Source: CAD feature listing. Evaluate the final solid. Frame: model axes, mm. Face numbers are marked on the shaded views. A direction names the side the tool comes from. Give positions to 0.01 mm unless a question says otherwise; leave off trailing zeros. Order: outer loops, then holes, each group sorted by start corner. A loop starts at its lowest first (then second) coordinate and runs counter-clockwise, first axis right, second up.
from build123d import *

# Parameters (mm, degrees)
SKETCH_1_R           = 3.5
EXTRUDE_1_DEPTH      = 43
SKETCH_2_OUTSIDE_W   = 17.824
SKETCH_2_OUTSIDE_H   = 17.824
SKETCH_2_OUTSIDE_W_2 = 10.593795304
SKETCH_2_OUTSIDE_H_2 = 5
CUT_EXTRUDE_1_DEPTH  = 18.4
EXTRUDE_START        = -3.9
SKETCH_5_R           = 5
EXTRUDE_2_DEPTH      = 11.8
SKETCH_3_R           = 1.175
CUT_EXTRUDE_2_DEPTH  = 1
SKETCH_6_R           = 1.15
CUT_EXTRUDE_3_DEPTH  = 6


with BuildPart() as part:
    # 草图1 → 凸台-拉伸1 (new body)
    with BuildSketch(Plane.XY):
        Circle(SKETCH_1_R)
    extrude(amount=EXTRUDE_1_DEPTH)

    # 草图2 outside → 切除-拉伸1 (cut)
    with BuildSketch(Plane.XY.offset(43)):
        Rectangle(SKETCH_2_OUTSIDE_W, SKETCH_2_OUTSIDE_H)
        Rectangle(SKETCH_2_OUTSIDE_W_2, SKETCH_2_OUTSIDE_H_2, mode=Mode.SUBTRACT)
    extrude(amount=-CUT_EXTRUDE_1_DEPTH, mode=Mode.SUBTRACT)

    # 草图5 → 凸台-拉伸2 (add)
    with BuildSketch(Plane(origin=(0, 0, 0), x_dir=(-1, 0, 0), z_dir=(0, 0, -1)).offset(EXTRUDE_START)):
        Circle(SKETCH_5_R)
    extrude(amount=-EXTRUDE_2_DEPTH)

    # 草图3 → 切除-拉伸2 (cut)
    with BuildSketch(Plane.XY.offset(43)):
        Circle(SKETCH_3_R)
    extrude(amount=-CUT_EXTRUDE_2_DEPTH, mode=Mode.SUBTRACT)

    # 草图6 → 切除-拉伸3 (cut)
    with BuildSketch(Plane.XY.offset(42)):
        Circle(SKETCH_6_R)
    extrude(amount=-CUT_EXTRUDE_3_DEPTH, mode=Mode.SUBTRACT)


solid = part.part
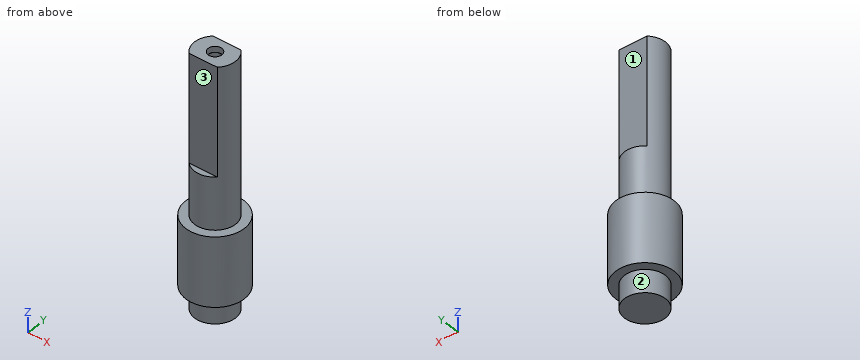
1) Section query C-C on x = 0. Output: boundary loops of the cut face in (y, z) (3 decimals), and give its area (3 significant figures).
Checks:
outline: (-5, 3.9) - (-3.5, 3.9) - (-3.5, 0) - (3.5, 0) - (3.5, 3.9) - (5, 3.9) - (5, 15.7) - (3.5, 15.7) - (3.5, 24.6) - (2.5, 24.6) - (2.5, 43) - (1.175, 43) - (1.175, 42) - (1.15, 42) - (1.15, 36) - (-1.15, 36) - (-1.15, 42) - (-1.175, 42) - (-1.175, 43) - (-2.5, 43) - (-2.5, 24.6) - (-3.5, 24.6) - (-3.5, 15.7) - (-5, 15.7) - close
area: 283 mm2
2) First-contact query: pin 1 Ø1 at (x, z) = (3.5, 12.5) entering from +Y; pin 2 Ø1 at (x, z) = (-2, 12.5) entering from -Y; pin 3 Ø2.5 at (x, z) = (-0.5, 32.5) entering from +Y. Flat tips, straight axial feed; report the tip coordinate or a pass-through.
Checks:
pin 1: stops at y = 4
pin 2: stops at y = -4.77
pin 3: stops at y = 2.5
3) Ray query, L1, parallel to Z at x = 0.25, y = 0; L2, parallel to Y at x = 0, z = 42.35 (3 decimals); L3, parallel to Y at x = -1.25, z = 29. Return the intervals inside material, ascending.
Checks:
L1: z = 0 to 36
L2: y = -2.5 to -1.175, 1.175 to 2.5
L3: y = -2.5 to 2.5
4) Reachability of the marked faces 1, 2 and 3 from +Z, -Z, +X, -X, +Y, -Y: full face, straight path, thin tool, end or side. Return the list, or none.
Checks:
face 1: +Z, +X, -X, +Y
face 2: -Z
face 3: +Z, +X, -X, -Y
5) Section query D-D on z = 5.5. Output: boundary loops of the cut face in (x, y).
Checks:
outline: circle Ø10 at (0, 0)
6) Section query B-B on y = 0. Output: boundary loops of the cut face in (x, z) (3 decimals), and give its area (3 significant figures).
Checks:
outline: (-5, 3.9) - (-3.5, 3.9) - (-3.5, 0) - (3.5, 0) - (3.5, 3.9) - (5, 3.9) - (5, 15.7) - (3.5, 15.7) - (3.5, 43) - (1.175, 43) - (1.175, 42) - (1.15, 42) - (1.15, 36) - (-1.15, 36) - (-1.15, 42) - (-1.175, 42) - (-1.175, 43) - (-3.5, 43) - (-3.5, 15.7) - (-5, 15.7) - close
area: 320 mm2
7) Section query A-A on z = 40.5. Output: boundary loops of the cut face in (x, y), and give its area (3 significant figures).
Checks:
outline: (-2.45, -2.5) - (2.45, -2.5) arc R3.5 ccw to (2.45, 2.5) - (-2.45, 2.5) arc R3.5 ccw to start; hole circle Ø2.3 at (0, 0)
area: 27.6 mm2
